from build123d import *

# Parameters (mm, degrees)
SKETCH1_W             = 25.4
SKETCH1_H             = 25.4
BOSS_EXTRUDE1_DEPTH   = 254
BOSS_EXTRUDE1_2_DEPTH = 254
SKETCH2_W             = 558.8
SKETCH2_H             = 25.4
BOSS_EXTRUDE2_DEPTH   = 25.4
BOSS_EXTRUDE3_DEPTH   = 25.4
BOSS_EXTRUDE4_DEPTH   = 25.4


with BuildPart() as part:
    # Sketch1 → Boss-Extrude1 (new, symmetric)
    with BuildSketch(Plane(origin=(0, 0, 0), x_dir=(1, 0, 0), z_dir=(0, 1, 0))):
        with Locations((12.7, 12.7)):
            Rectangle(SKETCH1_W, SKETCH1_H)
    extrude(amount=BOSS_EXTRUDE1_DEPTH, both=True)



with BuildPart() as body_2:
    # Sketch1 → Boss-Extrude1 2 (new, symmetric)
    with BuildSketch(Plane(origin=(0, 0, 0), x_dir=(1, 0, 0), z_dir=(0, 1, 0))):
        with Locations((596.9, 12.7)):
            Rectangle(SKETCH1_W, SKETCH1_H)
    extrude(amount=BOSS_EXTRUDE1_2_DEPTH, both=True)


with BuildPart() as part_1:
    add(part.part)

    add(body_2.part)  # Boss-Extrude2 merges body 2
    # Sketch2 → Boss-Extrude2 (add)
    with BuildSketch(Plane(origin=(0, 254, 0), x_dir=(1, 0, 0), z_dir=(0, 1, 0))):
        Polygon((0, 304.8), (0, 25.4), (25.4, 25.4), (25.4, 279.4), (584.2, 279.4), (584.2, 25.4), (609.6, 25.4), (609.6, 304.8), align=None)
        with Locations((304.8, 12.7)):
            Rectangle(SKETCH2_W, SKETCH2_H)
    extrude(amount=-BOSS_EXTRUDE2_DEPTH)

    # Sketch3 → Boss-Extrude3 (add)
    with BuildSketch(Plane(origin=(609.6, 0, 0), x_dir=(0, 0, -1), z_dir=(1, 0, 0))):
        Polygon((25.4, 128.021616083), (25.4, 100.578383917), (304.8, 214.878383917), (304.8, 228.6), (271.258271797, 228.6), align=None)
    extrude(amount=-BOSS_EXTRUDE3_DEPTH)

    # Sketch4 → Boss-Extrude4 (add)
    with BuildSketch(Plane.ZY):
        Polygon((-271.258271797, 228.6), (-25.4, 128.021616083), (-25.4, 100.578383917), (-304.8, 214.878383917), (-304.8, 228.6), align=None)
    extrude(amount=-BOSS_EXTRUDE4_DEPTH)


solid = part_1.part
Read the model definition and answer for the solid it produces. Units are mm, in the model's axes. A direction names the side the tool comes from. Give positions to 0.01 mm unless a question says otherwise; leave off trailing zeros. Write each loop counter-clockwise with the first axis right and the second up, starting at its lowest first coordinate (ties: lowest second). Pieces come first, ordered by that corner, then holes. Notation, with made-up numbers: (55.5, -22) -> (112.5, -22) arc R23 ccw to (112.5, -12) -> close; hole circle Ø7 at (26.5, -16.5). An arc over 180 degrees is marked (long way). Answer as a JSON object with one key per item and string values. Group by question number.
1) Find section B-B (y = 82.5). Write down the section's boundary in (x, z).
2) A tool of negligible diameter and unlimited length cuts with its end or side. For faces 5 (the flat face through (597, 228.6, -150)), 6 (the flat face through (301, 228.6, -13)), 7 (the flat face through (13, -74, -25.4)), 8 (the flat face through (301, 241, -25.4)), from which of +Z, -Z, +X, -X, +Y, -Y can it reach the whole face along a straight path? Write none if from no direction.
3) Find section A-A (x = 553). Write down the section's boundary in (y, z), and give its area (3 significant figures).
4) Find section D-D (z = -69.5). Write down the section's boundary in (x, y), and give its area (3 significant figures).
5) Find section C-C (y = 169.5). Write down the section's boundary in (x, z), and give its area (3 significant figures).
6) Consider L1, parallel to X at y = 21, z = -18; L2, parallel to Y at x = 547, z = -23.5. Determine where each line is inside the solid, lowest interval first. Write a range as from..to.
7) Each of these flat-tipped pins is pushed along its axis until it touches: P1, Ø12.5, axis at x = 14.5, z = -194, coming from the -Y side; P2, Ø7.5, axis at x = 178.5, z = -18, coming from the -Y side; P3, Ø12.5, axis at x = 595.5, y = -81, coming from the -Z side. Where does it stop, or does it pass through?
8) The mould has two halves that part along Z. Classify faces 1 (the flat face through (301, 241, -279.4)), 2 (the flat face through (597.078, 156.928, -163.144)), 3 (the flat face through (584.2, 133, -84)), 4 (the flat face through (597, -254, -13)): +Z half, -Z half, draft (parallel to the pull), parting line (faces both ways), or undercut.
Values follow:
{
 "1": {"outline": "(0, -25.4) -> (25.4, -25.4) -> (25.4, 0) -> (0, 0) -> close; (584.2, -25.4) -> (609.6, -25.4) -> (609.6, 0) -> (584.2, 0) -> close"},
 "2": {"face 5": "+X, -X", "face 6": "+Z, -Z, -Y", "face 7": "-Z, +X, -X, -Y", "face 8": "+Y, -Y"},
 "3": {"outline": "(228.6, -304.8) -> (254, -304.8) -> (254, -279.4) -> (228.6, -279.4) -> close; (228.6, -25.4) -> (254, -25.4) -> (254, 0) -> (228.6, 0) -> close", "area": "1,290 mm2"},
 "4": {"outline": "(0, 118.62) -> (25.4, 118.62) -> (25.4, 146.06) -> (0, 146.06) -> close; (0, 228.6) -> (25.4, 228.6) -> (25.4, 254) -> (0, 254) -> close; (584.2, 118.62) -> (609.6, 118.62) -> (609.6, 146.06) -> (584.2, 146.06) -> close; (584.2, 228.6) -> (609.6, 228.6) -> (609.6, 254) -> (584.2, 254) -> close", "area": "2,680 mm2"},
 "5": {"outline": "(0, -193.88) -> (25.4, -193.88) -> (25.4, -126.79) -> (0, -126.79) -> close; (0, -25.4) -> (25.4, -25.4) -> (25.4, 0) -> (0, 0) -> close; (584.2, -193.88) -> (609.6, -193.88) -> (609.6, -126.79) -> (584.2, -126.79) -> close; (584.2, -25.4) -> (609.6, -25.4) -> (609.6, 0) -> (584.2, 0) -> close", "area": "4,700 mm2"},
 "6": {"L1": "x = 0..25.4, 584.2..609.6", "L2": "y = 228.6..254"},
 "7": {"P1": "stops at y = 166.99", "P2": "stops at y = 228.6", "P3": "stops at z = -25.4"},
 "8": {"face 1": "undercut", "face 2": "-Z half", "face 3": "undercut", "face 4": "draft"}
}
